from build123d import *

# Parameters (mm, degrees)
BOSS_EXTRU_1_DEPTH = 150
ESQUISSE2_W        = 400
ESQUISSE2_H        = 110
BOSS_EXTRU_2_DEPTH = 30


with BuildPart() as part:
    # Esquisse1 → Boss.-Extru.1 (new body)
    with BuildSketch(Plane(origin=(0, 0, 0), x_dir=(0, 0, -1), z_dir=(1, 0, 0))):
        Polygon((0, 80), (0, 0), (30, 0), (30, 110), (-370, 110), (-370, 0), (-340, 0), (-340, 80), align=None)
    extrude(amount=BOSS_EXTRU_1_DEPTH)

    # Esquisse2 → Boss.-Extru.2 (add)
    with BuildSketch(Plane.ZY):
        with Locations((170, 55)):
            Rectangle(ESQUISSE2_W, ESQUISSE2_H)
    extrude(amount=BOSS_EXTRU_2_DEPTH)


solid = part.part
For this review, take the finished solid that the model builds, in its own axes (mm). A direction names the side the tool comes from. Round coordinates to 2 decimals unless told otherwise and drop trailing zeros. Order: outer loops, then holes, each group sorted by start corner. A loop starts at its lowest first (then second) coordinate and runs counter-clockwise, first axis right, second up. Notation, with made-up numbers: (-32.75, 6) -> (0.25, 6) arc R8 cw to (0.25, 19) -> close; hole circle Ø11 at (76.25, 0.5). An arc over 180 degrees is marked (long way). Put each result on its own line as item: value.
Q1. Insertion check: pin 1 Ø8 at (y, z) = (70.5, 306) entering from +X. The pin has a flat end and moves straight along its axis. Give the tip position at first contact, or say it passes through.
Check result:
pin 1: x = 0
Q2. Machinability: for faces 1 (the flat face through (61, 54, -30)), 2 (the flat face through (74, 39, 340)), which of the approach directions +Z, -Z, +X, -X, +Y, -Y give a long, thin tool a straight path to every point of the face, cutting with its end or side? Answer none if there is none.
Check result:
face 1: -Z, +X, -X, +Y, -Y
face 2: +X, -Y
Q3. Add section B-B on z = 77. Write out the cut boundary in (x, y), plus the area to 3 significant figures.
Check result:
outline: (-30, 0) -> (0, 0) -> (0, 80) -> (150, 80) -> (150, 110) -> (-30, 110) -> close
area: 7,800 mm2
Q4. Add section C-C on y = 33. Write out the cut boundary in (x, z), plus the area to 3 significant figures.
Check result:
outline: (-30, -30) -> (150, -30) -> (150, 0) -> (0, 0) -> (0, 340) -> (150, 340) -> (150, 370) -> (-30, 370) -> close
area: 21,000 mm2
Q5. For probe 1 along Z at (x, y) = (19, 73); probe 2 along X at (y, z) = (8, 9); probe 3 along Y at (x, z) = (84, 157.5), list the stretches that pass through material, from the lowest coordinate up. Write a range as [from, to].
Check result:
probe 1: [-30, 0], [340, 370]
probe 2: [-30, 0]
probe 3: [80, 110]
Q6. Mouldability with a two-part tool opening along Z and no side actions: class faces 3 (the flat face through (-30, 56, 167)), 4 (the flat face through (61, 54, 370)), 5 (the flat face through (0, 41, 168)) as pulls with the +Z half, pulls with the -Z half, needs draft (parallel to the pull), parting line crosses it, or undercut.
Check result:
face 3: needs draft
face 4: pulls with the +Z half
face 5: undercut
Q7. Add section A-A on x = 74. Write out the cut boundary in (y, z), plus the area to 3 significant figures.
Check result:
outline: (0, -30) -> (110, -30) -> (110, 370) -> (0, 370) -> (0, 340) -> (80, 340) -> (80, 0) -> (0, 0) -> close
area: 16,800 mm2
